Geometry: see drawing. Coordinates: mm, zero at the bounding-box minimum. Give positions to 0.01 mm unless a question says otherwise; leave off trailing zeros. Write each loop counter-clockwise with the first axis right and the second up, starting at its lowest first coordinate (ties: lowest second). Pieces come first, ordered by that corner, then holes. Notation, with made-up numbers: (-4, -2.5) - (13, -2.5) arc R26 ccw to (13, 23.5) - close; hole circle Ø9 at (15.25, 2.25). An arc over 180 degrees is marked (long way). Use a Markdown table: item, result. Add a question column.
1. Material intervals for probe 1 along X at (y, z) = (2.75, 9.5); probe 2 along X at (y, z) = (2.5, 10); probe 3 along Z at (x, y) = (288.48, 3), sorted ascending.
2. Section query A-A, the plane z = 16.52. Return loops of the section in (x, y).
3. Section query C-C, the plane x = 288.48. Return loops of the section in (y, z), plus the area to 3 significant figures.
4. Section query B-B, the plane z = 32.5. Return loops of the section in (x, y).
5. Pin query (flat end, axial travel): pin 1 (2 mm diameter, centred on y = 4.5, z = 58, fed in from -X); pin 2 (4 mm diameter, centred on x = 288.48, z = 48.48, fed in from -Y). Return the tip coordinate at first contact, or that it passes through.
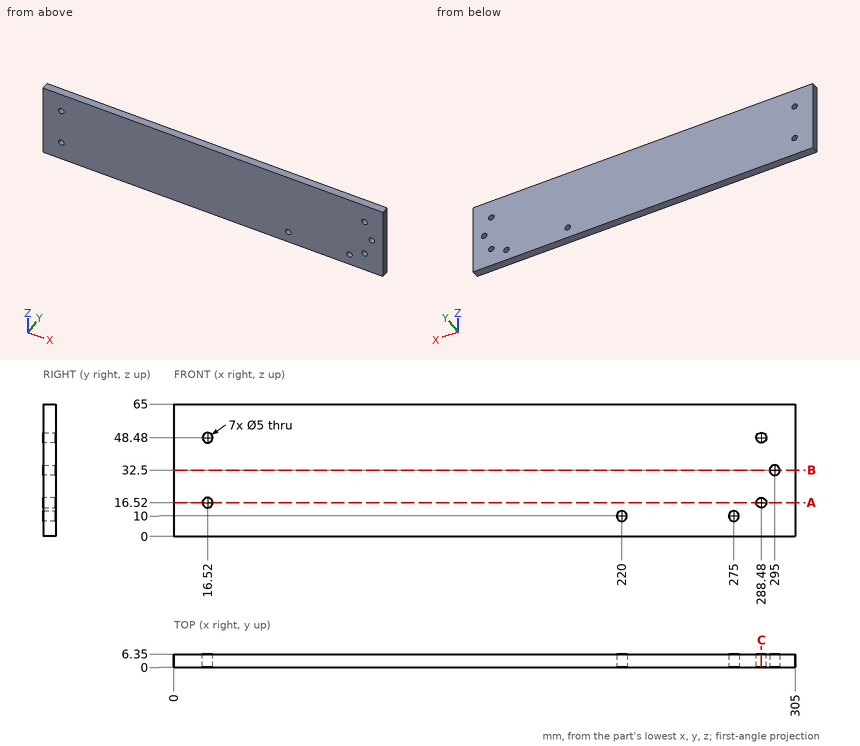
Result sheet:
| question | item | result |
|---|---|---|
| 1 | probe 1 | x = 0 to 217.55, 222.45 to 272.55, 277.45 to 305 |
| 1 | probe 2 | x = 0 to 217.5, 222.5 to 272.5, 277.5 to 305 |
| 1 | probe 3 | z = 0 to 14.02, 19.02 to 45.98, 50.98 to 65 |
| 2 | outline | (0, 0) - (14.02, 0) - (14.02, 6.35) - (0, 6.35) - close; (19.02, 0) - (285.98, 0) - (285.98, 6.35) - (19.02, 6.35) - close; (290.98, 0) - (305, 0) - (305, 6.35) - (290.98, 6.35) - close |
| 3 | outline | (0, 0) - (6.35, 0) - (6.35, 14.02) - (0, 14.02) - close; (0, 19.02) - (6.35, 19.02) - (6.35, 45.98) - (0, 45.98) - close; (0, 50.98) - (6.35, 50.98) - (6.35, 65) - (0, 65) - close |
| 3 | area | 349 mm² |
| 4 | outline | (0, 0) - (292.5, 0) - (292.5, 6.35) - (0, 6.35) - close; (297.5, 0) - (305, 0) - (305, 6.35) - (297.5, 6.35) - close |
| 5 | pin 1 | stops at x = 0 |
| 5 | pin 2 | passes through |
